Part print with two shaded views. Sizes in mm from the minimum x, y, z corner. A direction names the side the tool comes from. Coordinates: 2 decimals unless noted, no trailing zeros. Loops run counter-clockwise (first coordinate to the right, second up) from the corner with the lowest first, then second, coordinate; pieces in that order, holes last. Notation, with made-up numbers: (2, 85.25) - (54, 85.25) arc R20 ccw to (54, 105.25) - close; hole circle Ø8 at (-34, 47). An arc over 180 degrees is marked (long way). Write each question's results on one line, items separated by ' | '. Start each with the question number.
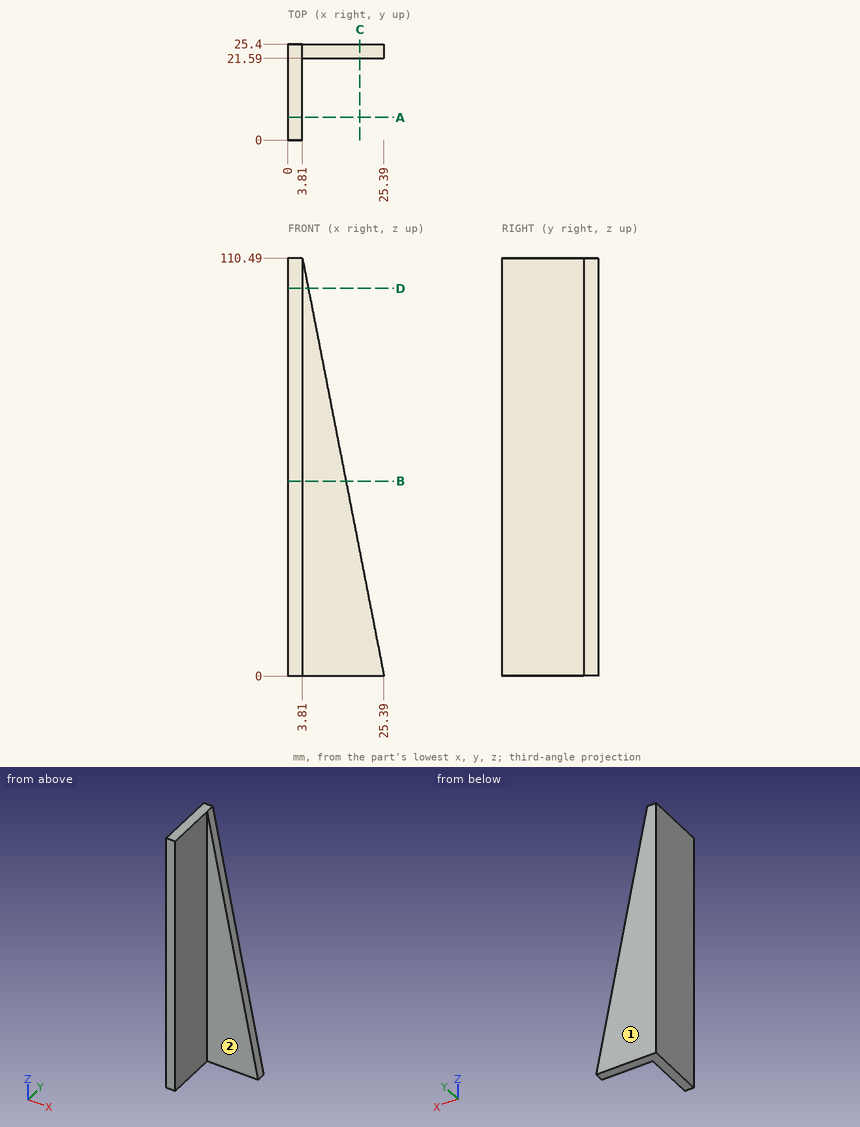
Q1. Which spindle directions (+Z, -Z, +X, -X, +Y, -Y) get a long thin tool onto all of the face, cutting with end or side? Do the marked faces 1 and 2. Say none if no direction does.
Q2. Pin check, flat tips, straight feed: pin 1 (5 mm diameter, centred on x = 10.5, z = 41.5, fed in from -Y); pin 2 (5 mm diameter, centred on x = 7.5, y = 13, fed in from -Z); pin 3 (5 mm diameter, centred on y = 7.5, z = 83, fed in from +X). Stop position of each tip, or through.
Q3. Cut at B-B (z = 51.5). List the corners of the cut face in (x, y), and give its area (3 significant figures).
Q4. Drill centre lines: L1, parallel to Y at x = 8.5, z = 36.5; L2, parallel to X at y = 4.25, z = 85; L3, parallel to X at y = 23.25, z = 7.5 (1 decimal). Where is each one in solid material? Low to high. Write a range as from..to.
Q5. Cut at C-C (x = 19). List the corners of the cut face in (y, z), and give its area (3 significant figures).
Q6. Cut at D-D (z = 102.5). List the corners of the cut face in (x, y).
Q7. Cut at A-A (y = 6). List the corners of the cut face in (x, z), and give its area (3 significant figures).
Check result:
1) face 1: +Z, -Z, +X, -X, +Y | face 2: +Z, -Z, +X, -Y
2) pin 1: y = 21.59 | pin 2: through | pin 3: x = 3.81
3) outline: (0, 0) - (3.81, 0) - (3.81, 21.59) - (15.33, 21.59) - (15.33, 25.4) - (0, 25.4) - close | area: 141 mm²
4) L1: 21.59..25.4 | L2: 0..3.81 | L3: 0..23.9
5) outline: (21.59, 0) - (25.4, 0) - (25.4, 32.72) - (21.59, 32.72) - close | area: 125 mm²
6) outline: (0, 0) - (3.81, 0) - (3.81, 21.59) - (5.37, 21.59) - (5.37, 25.4) - (0, 25.4) - close
7) outline: (0, 0) - (3.81, 0) - (3.81, 110.49) - (0, 110.49) - close | area: 421 mm²
